Design review of the part built by this model. Coordinates are the model's own, in mm. Face numbers are marked on the shaded views. A direction names the side the tool comes from. Give positions to 0.01 mm unless a question says otherwise; leave off trailing zeros. Order: outer loops, then holes, each group sorted by start corner. A loop starts at its lowest first (then second) coordinate and runs counter-clockwise, first axis right, second up. Notation, with made-up numbers: (70, -23.5) - (107, -23.5) arc R18 cw to (107, 11.5) - close; hole circle Ø5 at (61, 42). An arc over 180 degrees is marked (long way). Write each question's results on one line, items separated by ' | '. Start each with the question number.
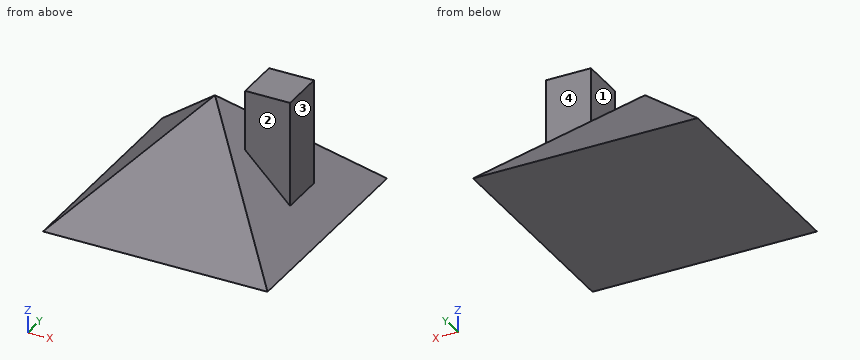
```python
from build123d import *

# Parameters (mm, degrees)
F0_W        = 63.5
F0_H        = 63.5
F0_W_2      = 12.7
F0_H_2      = 12.7
F1_DEPTH    = 31.75
F2_T1_DEPTH = 226.8018697358
F2_T3_DEPTH = 226.8018697358
F3_DEPTH    = 38.1


# Not quite as in the source:
# - a fillet or chamfer that OpenCascade refuses, or shapes differently, is made with other operations: its cross-section is extruded or revolved along the edge and cut away or added


with BuildPart() as f1:
    # F0 (on Top) → F1 (new body)
    with BuildSketch(Plane.XY):
        with Locations((0.9875343293, -0.9437446371)):
            Rectangle(F0_W, F0_H)
        with Locations((18.0756017402, 1.2459141038)):
            Rectangle(F0_W_2, F0_H_2, mode=Mode.SUBTRACT)
    extrude(amount=F1_DEPTH)

    # F2: chamfer of 31.75 on 4 edges, made by hand

    # F2_s2 → F2_t1 (cut)
    with BuildSketch(Plane.YZ.offset(-112.4134005386)):
        Polygon((-32.6937446371, 0), (-0.9437446371, 31.75), (-32.6937446371, 31.75), align=None)
        Polygon((30.8062553629, 0), (-0.9437446371, 31.75), (30.8062553629, 31.75), align=None)
    extrude(amount=F2_T1_DEPTH, mode=Mode.SUBTRACT)

    # F2_s4 → F2_t3 (cut)
    with BuildSketch(Plane.XZ.offset(-112.4571902308)):
        Polygon((32.7375343293, 0), (0.9875343293, 31.75), (32.7375343293, 31.75), align=None)
        Polygon((-30.7624656707, 0), (0.9875343293, 31.75), (-30.7624656707, 31.75), align=None)
    extrude(amount=F2_T3_DEPTH, mode=Mode.SUBTRACT)

    # F0 (on Top) → F3 (join)
    with BuildSketch(Plane.XY):
        with Locations((18.0756017402, 1.2459141038)):
            Rectangle(F0_W_2, F0_H_2)
    extrude(amount=F3_DEPTH)


solid = f1.part
```
Q1. Insertion check: pin 1 Ø1 at (y, z) = (-7.5, 9) entering from -X; pin 2 Ø4 at (x, z) = (20, 27) entering from +Y; pin 3 Ø4 at (y, z) = (-11.5, 5.5) entering from +X. Each pin has a flat end and moves straight along its axis. Give the tip position at first contact, or say it passes through.
Q2. Add section C-C (z = 13.5). Give the boundary of the cut face in (x, y), plus the area to 3 significant figures.
Q3. Machinability: for the marked faces 1, 2, 3 and 4, which of the approach directions +Z, -Z, +X, -X, +Y, -Y give a long, thin tool a straight path to every point of the face, cutting with its end or side? Answer none if there is none.
Q4. For line 1 (Y direction, x = 16.5, z = 36.5); line 2 (X direction, y = -2.5, z = 32.5); line 3 (Z direction, x = -15, y = 18.5), list the stretches that pass through material, from the lowest coordinate up. Write a range as [from, to].
Q5. Add section B-B (x = 14.5). Give the boundary of the cut face in (y, z).
Q6. Add section D-D (y = -14.5). Give the boundary of the cut face in (x, z).
Q7. Add section A-A (z = 24). Give the boundary of the cut face in (x, y).
Verdict:
1) pin 1: stops at x = -22.26 | pin 2: stops at y = 7.6 | pin 3: stops at x = 29.24
2) outline: (-17.26, -19.19) - (19.24, -19.19) - (19.24, -5.1) - (24.43, -5.1) - (24.43, 7.6) - (19.24, 7.6) - (19.24, 17.31) - (-17.26, 17.31) - close | area: 1,400 mm2
3) face 1: +Z, +Y, -Y | face 2: +Z, +X, -Y | face 3: +Z, +X, +Y, -Y | face 4: +Z, +X, +Y
4) line 1: y = [-5.1, 7.6] | line 2: x = [11.73, 24.43] | line 3: z = [0, 12.31]
5) outline: (-32.69, 0) - (30.81, 0) - (12.57, 18.24) - (7.6, 18.24) - (7.6, 38.1) - (-5.1, 38.1) - (-5.1, 18.24) - (-14.46, 18.24) - close
6) outline: (-30.76, 0) - (32.74, 0) - (14.54, 18.19) - (-12.57, 18.19) - close
7) outline: (-6.76, -8.69) - (8.74, -8.69) - (8.74, 6.81) - (-6.76, 6.81) - close; (11.73, -5.1) - (24.43, -5.1) - (24.43, 7.6) - (11.73, 7.6) - close
